from build123d import *

# Parameters (mm, degrees)
F0_R     = 76.2
F0_R_2   = 50.8
F1_DEPTH = 127
F3_DEPTH = 25.4
F4_W     = 304.8
F4_H     = 50.8
F5_DEPTH = 152.4
F7_DEPTH = 76.2


with BuildPart() as f1:
    # F0 (on Front) → F1 (new body)
    with BuildSketch(Plane.XZ):
        Circle(F0_R)
        Circle(F0_R_2, mode=Mode.SUBTRACT)
    extrude(amount=F1_DEPTH)

    # F2 (on Front) → F3 (join)
    with BuildSketch(Plane.XZ):
        with BuildLine():
            ThreePointArc((0, -76.2), (-62.1944082776, -44.0260783968), (-71.8681337184, 25.3261002888))
            Line((-71.8681337184, 25.3261002888), (-152.4, -203.2))
            Line((-152.4, -203.2), (0, -203.2))
            Line((0, -203.2), (0, -76.2))
        make_face()
        with BuildLine():
            ThreePointArc((71.8681337184, 25.3261002888), (62.1944082776, -44.0260783968), (0, -76.2))
            Line((0, -76.2), (0, -203.2))
            Line((0, -203.2), (152.4, -203.2))
            Line((152.4, -203.2), (71.8681337184, 25.3261002888))
        make_face()
    extrude(amount=F3_DEPTH)

    # F4 (on face) → F5 (join)
    with BuildSketch(Plane(origin=(0, 0, 0), x_dir=(-1, 0, 0), z_dir=(0, 1, 0))):
        with Locations((0, -228.6)):
            Rectangle(F4_W, F4_H)
    extrude(amount=-F5_DEPTH)

    # F6 (on face) → F7 (join)
    with BuildSketch(Plane.XZ.offset(25.4)):
        with BuildLine():
            Line((0, -203.2), (0, -76.2))
            ThreePointArc((0, -76.2), (-6.3723210333, -75.9330858365), (-12.7, -75.1342132454))
            Line((-12.7, -75.1342132454), (-12.7, -203.2))
            Line((-12.7, -203.2), (0, -203.2))
        make_face()
        with BuildLine():
            ThreePointArc((12.7, -75.1342132454), (6.3723210333, -75.9330858365), (0, -76.2))
            Line((0, -76.2), (0, -203.2))
            Line((0, -203.2), (12.7, -203.2))
            Line((12.7, -203.2), (12.7, -75.1342132454))
        make_face()
    extrude(amount=F7_DEPTH)


solid = f1.part
Design review of the part built by this model. Coordinates are the model's own, in mm. A direction names the side the tool comes from. Coordinates: 2 decimals unless noted, no trailing zeros. Order: outer loops, then holes, each group sorted by start corner. A loop starts at its lowest first (then second) coordinate and runs counter-clockwise, first axis right, second up. Notation, with made-up numbers: (-13, 69.5) -> (37, 69.5) arc R22 ccw to (37, 107.5) -> close; hole circle Ø2 at (53, 81). An arc over 180 degrees is marked (long way). Use one line per item in the form item = value. Start each with the question number.
(1) Add section C-C on z = 9. State the section outline as (x, y) points.
(2) Add section B-B on x = 0. State the section outline as (y, z) points, plus the area to 3 significant figures.
(3) Add section A-A on y = -113.5. State the section outline as (x, z) points, plus the area to 3 significant figures.
(4) Insertion check: pin 1 (4 mm diameter, centred on x = -28, y = -31.5, fed in from +Z); pin 2 (3 mm diameter, centred on y = -69, z = 8.5, fed in from +X); pin 3 (5 mm diameter, centred on x = -10, z = -184, fed in from +Y); pin 4 (2 mm diameter, centred on y = -88, z = -163.5, fed in from -X). Each pin has a flat end and moves straight along its axis. Give the tip position at first contact, or say it passes through.
(5) For faces 4 (the flat face through (12.7, -63, -140)), 5 (the flat face through (-12.7, -63, -138)), 6 (the cylindrical face through (-9.92, -76.72, 75.55)), 7 (the flat face through (112.7, -12.52, -90.54)), list the 3-axis set-ups (+Z, -Z, +X, -X, +Y, -Y) from which the entire face can be reached by the end or side of a thin tool; tool diameter is ignored.
(6) Add section D-D on y = -83.5. State the section outline as (x, z) points, plus the area to 3 significant figures.
(7) For probe 1 along Z at (x, y) = (29.5, -122.5); probe 2 along Z at (x, y) = (3.5, -119); probe 3 along Z at (x, y) = (0, -49.5), list the stretches that pass through material, from the lowest coordinate up.
(8) The part is to be moulded in two halves that separate along Z. For faces 1 (the flat face through (16, -127, -50)), 2 (the flat face through (0, -101.6, -138)), 3 (the flat face through (-111.57, -12.52, -87.34)), say which applies: +Z half, -Z half, draft (parallel to the pull), parting line (faces both ways), or undercut.
Answer block:
q1.outline = (-77.62, -25.4) -> (-75.67, -25.4) -> (-75.67, -127) -> (-50, -127) -> (-50, 0) -> (-77.62, 0) -> close; (50, -127) -> (75.67, -127) -> (75.67, -25.4) -> (77.62, -25.4) -> (77.62, 0) -> (50, 0) -> close
q2.outline = (-152.4, -254) -> (0, -254) -> (0, -50.8) -> (-127, -50.8) -> (-127, -76.2) -> (-101.6, -76.2) -> (-101.6, -203.2) -> (-152.4, -203.2) -> close; (-127, 50.8) -> (0, 50.8) -> (0, 76.2) -> (-127, 76.2) -> close
q2.area = 27,100 mm²
q3.outline = (-152.4, -254) -> (152.4, -254) -> (152.4, -203.2) -> (-152.4, -203.2) -> close; circle Ø152.4 at (0, 0); hole circle Ø101.6 at (0, 0)
q3.area = 25,600 mm²
q4.pin_1 = 71.63
q4.pin_2 = 75.88
q4.pin_3 = 0
q4.pin_4 = -12.7
q5.face_4 = +X, -Y
q5.face_5 = -X, -Y
q5.face_6 = -Y
q5.face_7 = +Z, +X, +Y, -Y
q6.outline = (-152.4, -254) -> (152.4, -254) -> (152.4, -203.2) -> (12.7, -203.2) -> (12.7, -75.13) arc R76.2 ccw (long way) to (-12.7, -75.13) -> (-12.7, -203.2) -> (-152.4, -203.2) -> close; hole circle Ø101.6 at (0, 0)
q6.area = 28,900 mm²
q7.probe_1 = -254 to -203.2, -70.26 to -41.36, 41.36 to 70.26
q7.probe_2 = -254 to -203.2, -76.12 to -50.68, 50.68 to 76.12
q7.probe_3 = -254 to -50.8, 50.8 to 76.2
q8.face_1 = draft
q8.face_2 = undercut
q8.face_3 = +Z half
